Geometry check sheet. Reference: drawing and pictorial views, mm from the part's lowest x, y, z. Coordinates: 2 decimals unless noted, no trailing zeros. Loops run counter-clockwise (first coordinate to the right, second up) from the corner with the lowest first, then second, coordinate; pieces in that order, holes last. Notation, with made-up numbers: (46.5, 27) -> (92.5, 27) arc R29 ccw to (92.5, 56) -> close; hole circle Ø3 at (58, 81). An arc over 180 degrees is marked (long way). Answer as a JSON object with one key per item and string values. Group by question number.
Q1. Gauge pin test, flat ends, axial feed: pin 1 Ø6.5 at (x, y) = (37.5, 9.5) entering from +Z; pin 2 Ø3 at (x, y) = (8, 4.5) entering from +Z; pin 3 Ø1.4 at (x, y) = (30.5, 7) entering from -Z; pin 4 Ø1.9 at (x, z) = (32, 2.5) entering from -Y. Record the tip position at first contact, or that the pin passes through.
Q2. Scan lines: L1, parallel to Y at x = 26, z = 2.1; L2, parallel to Y at x = 29, z = 3.2; L3, parallel to Z at x = 41.5, y = 11.25. Record each from-to range of solid material in increasing order.
Q3. Cross-section at B-B on x = 32. Record the boundary of the cut face in (y, z).
Q4. Cross-section at D-D on y = 11.25. Record the boundary of the cut face in (x, z).
Q5. Release check for a two-part mould opening along X. For the marked faces 1 and 2 record: released by +X, released by -X, zero draft, split by the parting line, or undercut.
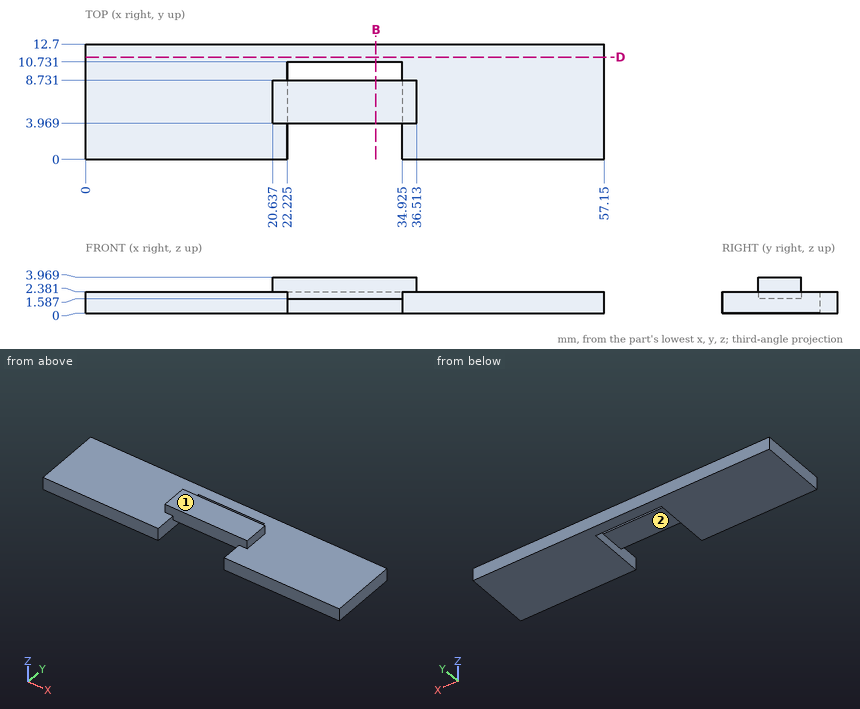
Computed values:
{
 "1": {"pin 1": "stops at z = 3.97", "pin 2": "stops at z = 2.38", "pin 3": "stops at z = 1.59", "pin 4": "stops at y = 3.97"},
 "2": {"L1": "y = 3.97 to 8.73, 10.73 to 12.7", "L2": "y = 3.97 to 8.73", "L3": "z = 0 to 2.38"},
 "3": {"outline": "(3.97, 1.59) -> (8.73, 1.59) -> (8.73, 3.97) -> (3.97, 3.97) -> close; (10.73, 0) -> (12.7, 0) -> (12.7, 2.38) -> (10.73, 2.38) -> close"},
 "4": {"outline": "(0, 0) -> (57.15, 0) -> (57.15, 2.38) -> (0, 2.38) -> close"},
 "5": {"face 1": "zero draft", "face 2": "undercut"}
}
